from build123d import *

# Parameters (mm, degrees)
SKETCH_1_W             = 60
SKETCH_1_H             = 60
EXTRUDE_1_DEPTH        = 8
HOLE_WIZARD_1_D        = 3
HOLE_WIZARD_2_D        = 5
HOLE_WIZARD_2_DEPTH    = 3
SKETCH_9_W             = 25
SKETCH_9_H             = 60
EXTRUDE_2_DEPTH        = 8
SKETCH_10_W            = 4
SKETCH_10_H            = 60
EXTRUDE_3_DEPTH        = 20
FILLET_1_R             = 5
SKETCH_11_W            = 100
SKETCH_11_H            = 60
EXTRUDE_4_DEPTH        = 8
SKETCH_17_W            = 180
SKETCH_17_H            = 60
EXTRUDE_5_DEPTH        = 8
HOLE_WIZARD_3_D        = 3
HOLE_WIZARD_4_D        = 5
HOLE_WIZARD_4_DEPTH    = 3
HOLE_WIZARD_5_D        = 3.5
HOLE_WIZARD_6_D        = 6.5
HOLE_WIZARD_6_DEPTH    = 4
SKETCH_25_W            = 104
SKETCH_25_H            = 60
EXTRUDE_7_DEPTH        = 36
SKETCH_26_W            = 100
SKETCH_26_H            = 52.5
CUT_EXTRUDE_1_DEPTH    = 36
SKETCH_27_W            = 8
SKETCH_27_H            = 60
EXTRUDE_8_DEPTH        = 10
HOLE_WIZARD_7_D        = 3.5
HOLE_WIZARD_7_DEPTH    = 10
FILLET_2_R             = 3
HOLE_WIZARD_8_D        = 2.5
HOLE_WIZARD_9_D        = 4.2
HOLE_WIZARD_9_DEPTH    = 4
SKETCH_37_W            = 30
SKETCH_37_H            = 60
CUT_EXTRUDE_2_DEPTH    = 174.481987538
FILLET_3_R             = 4
HOLE_WIZARD_10_D       = 3.5
PATTERN_LINEAR_1_COUNT = 6
PATTERN_LINEAR_1_PITCH = 10
HOLE_WIZARD_11_D       = 6
HOLE_WIZARD_11_DEPTH   = 4
PATTERN_LINEAR_2_COUNT = 6
PATTERN_LINEAR_2_PITCH = 10
HOLE_WIZARD_12_D       = 3.5
HOLE_WIZARD_13_D       = 6
HOLE_WIZARD_13_DEPTH   = 4
EXTRUDE_9_DEPTH        = 8
EXTRUDE_10_DEPTH       = 4
HOLE_WIZARD_14_D       = 3.5


with BuildPart() as part:
    # 草图1 → 凸台-拉伸1 (new body)
    with BuildSketch(Plane.XY):
        with Locations((30, 30)):
            Rectangle(SKETCH_1_W, SKETCH_1_H)
    extrude(amount=EXTRUDE_1_DEPTH)

    # 孔1 (through all)
    with Locations(Plane(origin=(0, 0, 0), x_dir=(-1, 0, 0), z_dir=(0, 0, -1))):
        with Locations((-51.5, 51.5), (-8.5, 51.5), (-8.5, 8.5), (-51.5, 8.5)):
            Hole(HOLE_WIZARD_1_D / 2)

    # 孔2
    with Locations(Plane(origin=(0, 0, 0), x_dir=(-1, 0, 0), z_dir=(0, 0, -1))):
        with Locations((-51.5, 51.5), (-8.5, 51.5), (-8.5, 8.5), (-51.5, 8.5)):
            Hole(HOLE_WIZARD_2_D / 2, depth=HOLE_WIZARD_2_DEPTH)

    # 草图9 → 凸台-拉伸2 (add)
    with BuildSketch(Plane.XY.offset(8)):
        with Locations((-12.5, 30)):
            Rectangle(SKETCH_9_W, SKETCH_9_H)
    extrude(amount=-EXTRUDE_2_DEPTH)

    # 草图10 → 凸台-拉伸3 (add)
    with BuildSketch(Plane.XY.offset(8)):
        with Locations((-18, 30)):
            Rectangle(SKETCH_10_W, SKETCH_10_H)
    extrude(amount=EXTRUDE_3_DEPTH)

    # 圆角1
    fillet_1_edges = [part.edges().sort_by_distance(p)[0] for p in [
        (-16, 30, 8),
    ]]
    fillet(fillet_1_edges, radius=FILLET_1_R)

    # 草图11 → 凸台-拉伸4 (add)
    with BuildSketch(Plane.XY.offset(8)):
        with Locations((-70, 30)):
            Rectangle(SKETCH_11_W, SKETCH_11_H)
    extrude(amount=-EXTRUDE_4_DEPTH)

    # 草图17 → 凸台-拉伸5 (add)
    with BuildSketch(Plane.XY.offset(8)):
        with Locations((-30, 90)):
            Rectangle(SKETCH_17_W, SKETCH_17_H)
        with Locations((-30, -30)):
            Rectangle(SKETCH_17_W, SKETCH_17_H)
    extrude(amount=-EXTRUDE_5_DEPTH)

    # 孔3 (through all)
    with Locations(Plane.XY.offset(8)):
        with Locations((-106.5, 116.5), (-48.5, 116.5), (-48.5, 67.5), (-106.5, 67.5)):
            Hole(HOLE_WIZARD_3_D / 2)

    # 孔4
    with Locations(Plane(origin=(0, 0, 0), x_dir=(-1, 0, 0), z_dir=(0, 0, -1))):
        with Locations((48.5, 116.5), (106.5, 116.5), (106.5, 67.5), (48.5, 67.5)):
            Hole(HOLE_WIZARD_4_D / 2, depth=HOLE_WIZARD_4_DEPTH)

    # 孔5 (through all)
    with Locations(Plane.XY.offset(8)):
        with Locations((-114, -14.75), (-30, -14.75), (-30, -54.75), (-114, -54.75)):
            Hole(HOLE_WIZARD_5_D / 2)

    # 孔6
    with Locations(Plane(origin=(0, 0, 0), x_dir=(-1, 0, 0), z_dir=(0, 0, -1))):
        with Locations((30, -14.75), (114, -14.75), (114, -54.75), (30, -54.75)):
            Hole(HOLE_WIZARD_6_D / 2, depth=HOLE_WIZARD_6_DEPTH)

    # 草图25 → 凸台-拉伸7 (add)
    with BuildSketch(Plane.XY.offset(8)):
        with Locations((-68, 30)):
            Rectangle(SKETCH_25_W, SKETCH_25_H)
    extrude(amount=EXTRUDE_7_DEPTH)

    # 草图26 → 切除-拉伸1 (cut)
    with BuildSketch(Plane.XY.offset(44)):
        with Locations((-70, 30)):
            Rectangle(SKETCH_26_W, SKETCH_26_H)
    extrude(amount=-CUT_EXTRUDE_1_DEPTH, mode=Mode.SUBTRACT)

    # 草图27 → 凸台-拉伸8 (add)
    with BuildSketch(Plane.XY.offset(44)):
        Polygon((-33, 60), (-16, 60), (-8, 60), (-8, 68), (-33, 68), align=None)
        with Locations((-12, 30)):
            Rectangle(SKETCH_27_W, SKETCH_27_H)
        Polygon((-8, 0), (-16, 0), (-33, 0), (-33, -8), (-8, -8), align=None)
    extrude(amount=-EXTRUDE_8_DEPTH)

    # 孔7
    with Locations(Plane.XY.offset(44)):
        with Locations((-27, 64), (-12, 43), (-12, 17), (-27, -4)):
            Hole(HOLE_WIZARD_7_D / 2, depth=HOLE_WIZARD_7_DEPTH)

    # 圆角2
    fillet_2_edges = [part.edges().sort_by_distance(p)[0] for p in [
        (-33, 60, 39),
        (-33, 68, 39),
        (-8, 68, 39),
        (-8, -8, 39),
        (-33, -8, 39),
        (-33, 0, 39),
    ]]
    fillet(fillet_2_edges, radius=FILLET_2_R)

    # 孔8 (through all)
    with Locations(Plane.XY.offset(8)):
        with Locations((13, 108), (13, 72), (-23, 72), (-23, 108)):
            Hole(HOLE_WIZARD_8_D / 2)

    # 孔9
    with Locations(Plane(origin=(0, 0, 0), x_dir=(-1, 0, 0), z_dir=(0, 0, -1))):
        with Locations((-13, 108), (23, 108), (23, 72), (-13, 72)):
            Hole(HOLE_WIZARD_9_D / 2, depth=HOLE_WIZARD_9_DEPTH)

    # 草图37 → 切除-拉伸2 (cut, through all)
    with BuildSketch(Plane.XY.offset(8)):
        with Locations((45, 90)):
            Rectangle(SKETCH_37_W, SKETCH_37_H)
        with Locations((45, -30)):
            Rectangle(SKETCH_37_W, SKETCH_37_H)
    extrude(amount=-CUT_EXTRUDE_2_DEPTH, mode=Mode.SUBTRACT)

    # 圆角3
    fillet_3_edges = [part.edges().sort_by_distance(p)[0] for p in [
        (-120, 120, 4),
        (-120, -60, 4),
        (30, 60, 4),
        (30, 120, 4),
        (30, -60, 4),
        (30, 0, 4),
    ]]
    fillet(fillet_3_edges, radius=FILLET_3_R)

    # 孔10 (through all)
    with Locations(Plane.XY.offset(8)):
        with Locations((0, -55), (10, -55), (20, -55)):
            hole_wizard_10 = Hole(HOLE_WIZARD_10_D / 2)

    # 阵列(线性)1: 孔10 ×6, 2 skipped
    with Locations(*[(0, i * PATTERN_LINEAR_1_PITCH, 0) for i in range(1, PATTERN_LINEAR_1_COUNT) if i not in (3, 4)]):
        add(hole_wizard_10, mode=Mode.SUBTRACT)

    # 孔11
    with Locations(Plane(origin=(0, 0, 0), x_dir=(-1, 0, 0), z_dir=(0, 0, -1))):
        with Locations((0, -55), (-10, -55), (-20, -55)):
            hole_wizard_11 = Hole(HOLE_WIZARD_11_D / 2, depth=HOLE_WIZARD_11_DEPTH)

    # 阵列(线性)2: 孔11 ×6, 2 skipped
    with Locations(*[(0, i * PATTERN_LINEAR_2_PITCH, 0) for i in range(1, PATTERN_LINEAR_2_COUNT) if i not in (3, 4)]):
        add(hole_wizard_11, mode=Mode.SUBTRACT)

    # 孔12 (through all)
    with Locations(Plane.XY.offset(8)):
        with Locations((0, -21.5), (10, -21.5), (20, -21.5)):
            Hole(HOLE_WIZARD_12_D / 2)

    # 孔13
    with Locations(Plane(origin=(0, 0, 0), x_dir=(-1, 0, 0), z_dir=(0, 0, -1))):
        with Locations((-20, -21.5), (-10, -21.5), (0, -21.5)):
            Hole(HOLE_WIZARD_13_D / 2, depth=HOLE_WIZARD_13_DEPTH)

    # 草图48 → 凸台-拉伸9 (add)
    with BuildSketch(Plane.XY.offset(8)):
        Polygon((-45, 108), (-45, 104), (-41, 104), (-41, 112), (-45, 112), align=None)
        Polygon((-41, 80), (-45, 80), (-45, 76), (-45, 72), (-41, 72), align=None)
    extrude(amount=EXTRUDE_9_DEPTH)

    # 草图49 → 凸台-拉伸10 (add)
    with BuildSketch(Plane(origin=(-41, 0, 0), x_dir=(0, 0, -1), z_dir=(1, 0, 0))):
        Polygon((-16, 112), (-8, 120), (-8, 112), align=None)
        Polygon((-16, 104), (-8, 96), (-8, 104), align=None)
        Polygon((-16, 80), (-8, 88), (-8, 80), align=None)
        Polygon((-16, 72), (-8, 72), (-8, 64), align=None)
    extrude(amount=-EXTRUDE_10_DEPTH)

    # 孔14 (through all)
    with Locations(Plane(origin=(-41, 0, 0), x_dir=(0, 0, -1), z_dir=(1, 0, 0))):
        with Locations((-12, 108), (-12, 76)):
            Hole(HOLE_WIZARD_14_D / 2)


solid = part.part
The listing builds one solid part. Answer for the finished solid, in the listing's coordinates (mm). A direction names the side the tool comes from. Round coordinates to 2 decimals unless told otherwise and drop trailing zeros. Write each loop counter-clockwise with the first axis right and the second up, starting at its lowest first coordinate (ties: lowest second). Pieces come first, ordered by that corner, then holes. Notation, with made-up numbers: M 39,11.5 L 53,11.5 A28 cw 53,34.5 Z; hole C 35,80.5 d3. An arc over 180 degrees is marked long. Write each question's results on one line, items separated by ' | '. Start each with the question number.
(1) Determine the mould class of faces 1 (the flat face through (-41, 108, 10)), 2 (the cylindrical face through (17.79, -42.97, 2.03)), 3 (the flat face through (-46, -60, 4)), 4 (the cylindrical face through (17.6, -23.3, 2)) for opening direction X: +X half, -X half, draft (parallel to the pull), parting line (faces both ways), or undercut.
(2) Each of these flat-tipped pins is pushed along its axis until it touches: P1, Ø3, axis at x = -25, z = 39, coming from the -Y side; P2, Ø4, axis at x = 8.5, y = 8.5, coming from the +Z side; P3, Ø8, axis at y = 68, z = 11.5, coming from the +X side. Where does it stop, or does it pass through?
(3) The part is cut by section D-D, the plane y = 36. Write down the section's boundary in (x, z), and give its area (3 significant figures).
(4) Find the intervals of material crossed by line 1 (Y direction, x = -114, z = 3.15); line 2 (Y direction, x = 0, z = 5.35); line 3 (Y direction, x = -93, z = 34), in increasing order.
(5) The part is cut by section A-A, the plane z = 25. Write down the section's boundary in (x, y).
(6) The part is cut by section B-B, the plane y = 99. Write down the section's boundary in (x, z), and give its area (3 significant figures).
(7) The part is cut by section C-C, the plane x = 46.5. Write down the section's boundary in (y, z), and give its area (3 significant figures).
(8) For faces 5 (the flat face through (-8, 30, 39)), 6 (the flat face through (10, 7, 3)), 7 (the cylindrical face through (31.203, -1.141, 3.944)), determine the directions among +Z, -Z, +X, -X, +Y, -Y from which every point of the face is accessible in a straight line to the end or side of a thin tool.
Worked answers:
1) face 1: +X half | face 2: undercut | face 3: draft | face 4: undercut
2) P1: stops at y = -8 | P2: stops at z = 8 | P3: stops at x = 30
3) outline: M -120,0 L 60,0 L 60,8 L -11,8 A5 cw -16,13 L -16,34 L -8,34 L -8,44 L -20,44 L -20,8 L -120,8 Z | area: 1,670 mm²
4) line 1: y = -60 to -58, -51.5 to -18, -11.5 to 120 | line 2: y = -60 to -56.75, -53.25 to -46.75, -43.25 to -36.75, -33.25 to -23.25, -19.75 to -6.75, -3.25 to 120 | line 3: y = 0 to 3.75, 56.25 to 60
5) outline: M -120,0 L -16,0 L -16,60 L -120,60 L -120,56.25 L -20,56.25 L -20,3.75 L -120,3.75 Z
6) outline: M -120,0 L 30,0 L 30,8 L -41,8 L -41,11 L -45,11 L -45,8 L -120,8 Z | area: 1,210 mm²
7) outline: M 0,0 L 60,0 L 60,8 L 0,8 Z | area: 480 mm²
8) face 5: +Z, +X, +Y, -Y | face 6: -Z | face 7: +Z, -Z, +X, -Y
